from build123d import *

# Parameters (mm, degrees)
SKETCH_1_W          = 45
SKETCH_1_H          = 247
EXTRUDE_1_DEPTH     = 6
CUT_EXTRUDE_1_DEPTH = 249.095243808
M3X0_51_D           = 2.5
M3X0_51_DEPTH       = 8.5
M3X0_51_TIP         = 0.751075774
M3X0_52_D           = 2.5
M3X0_52_DEPTH       = 8.5
M3X0_52_TIP         = 0.751075774


with BuildPart() as part:
    # Эскиз1 → Бобышка-Вытянуть1 (new body)
    with BuildSketch(Plane(origin=(0, 0, 0), x_dir=(1, 0, 0), z_dir=(0, 1, 0))):
        with Locations((0, -123.5)):
            Rectangle(SKETCH_1_W, SKETCH_1_H)
    extrude(amount=EXTRUDE_1_DEPTH)

    # Эскиз2 → Вырез-Вытянуть1 (cut, through all)
    with BuildSketch(Plane(origin=(0, 6, 0), x_dir=(1, 0, 0), z_dir=(0, 1, 0))):
        with BuildLine():
            Line((-10.274368671, -73.5), (-10.274368671, -173.5))
            ThreePointArc((-10.274368671, -173.5), (-12.374368671, -175.6), (-14.474368671, -173.5))
            Line((-14.474368671, -173.5), (-14.474368671, -73.5))
            ThreePointArc((-14.474368671, -73.5), (-12.374368671, -71.4), (-10.274368671, -73.5))
        make_face()
        with BuildLine():
            Line((10.274368671, -73.5), (10.274368671, -173.5))
            ThreePointArc((10.274368671, -173.5), (12.374368671, -175.6), (14.474368671, -173.5))
            Line((14.474368671, -173.5), (14.474368671, -73.5))
            ThreePointArc((14.474368671, -73.5), (12.374368671, -71.4), (10.274368671, -73.5))
        make_face()
    extrude(amount=-CUT_EXTRUDE_1_DEPTH, mode=Mode.SUBTRACT)

    # Отверстие обработанное метчиком M3x0.51
    with Locations(Plane.XY.offset(247)):
        with Locations((-13.5, 3), (-4.5, 3), (4.5, 3), (13.5, 3)):
            Hole(M3X0_51_D / 2, depth=M3X0_51_DEPTH)
            with Locations((0, 0, -(M3X0_51_DEPTH + M3X0_51_TIP / 2))):  # 118° drill point
                Cone(0, M3X0_51_D / 2, M3X0_51_TIP, mode=Mode.SUBTRACT)

    # Отверстие обработанное метчиком M3x0.52
    with Locations(Plane(origin=(0, 0, 0), x_dir=(-1, 0, 0), z_dir=(0, 0, -1))):
        with Locations((-13.5, 3), (-4.5, 3), (4.5, 3), (13.5, 3)):
            Hole(M3X0_52_D / 2, depth=M3X0_52_DEPTH)
            with Locations((0, 0, -(M3X0_52_DEPTH + M3X0_52_TIP / 2))):  # 118° drill point
                Cone(0, M3X0_52_D / 2, M3X0_52_TIP, mode=Mode.SUBTRACT)


solid = part.part
Geometry: final body of the model. Coordinates: model frame, mm. A direction names the side the tool comes from. Round coordinates to 2 decimals unless told otherwise and drop trailing zeros. Loops run counter-clockwise (first coordinate to the right, second up) from the corner with the lowest first, then second, coordinate; pieces in that order, holes last. Notation, with made-up numbers: (89, 40.5) - (148, 40.5) arc R20 ccw to (148, 61.5) - close; hole circle Ø9 at (-5.5, -34.75). An arc over 180 degrees is marked (long way). Write each question's results on one line, items separated by ' | '. Start each with the question number.
1) Mould query, pull axis X, two halves, no side actions, for faces 1 (the face through (-14.474, 3, 124)), 2 (the face through (22.5, 3, 125)), 3 (the face through (-22.5, 3, 125)), 4 (the face through (0, 3, 0)). Classes: released by +X, released by -X, zero draft, split by the parting line, or undercut.
2) First-contact query: P1, Ø1.5, axis at x = -13.5, y = 3, coming from the -Z side; P2, Ø2, axis at x = -13.5, y = 3, coming from the -Z side; P3, Ø2, axis at x = -4.5, y = 3, coming from the +Z side. Flat tips, straight axial feed; report the tip coordinate or a pass-through.
3) Line query: probe 1 along X at (y, z) = (2.45, 144); probe 2 along X at (y, z) = (3, 6.25); probe 3 along Z at (x, y) = (-12, 4.8). Output: solid intervals per line, ascending. Write a range as [from, to].
4) Cut plane A-A on z = 149.5. Return loops of the section in (x, y), then the cut area to 3 significant figures.
5) Access query for faces 5 (the face through (14.474, 3, 124)), 6 (the face through (0, 0, 122)). Directions: +Z, -Z, +X, -X, +Y, -Y. A direction counts if a zero-diameter tool reaches every point of the face in a straight line with its end or side. Return the directions, or none.
Verdict:
1) face 1: undercut | face 2: released by +X | face 3: released by -X | face 4: zero draft
2) P1: stops at z = 8.8 | P2: stops at z = 8.65 | P3: stops at z = 238.35
3) probe 1: x = [-22.5, -14.47], [-10.27, 10.27], [14.47, 22.5] | probe 2: x = [-22.5, -14.75], [-12.25, -5.75], [-3.25, 3.25], [5.75, 12.25], [14.75, 22.5] | probe 3: z = [0, 71.43], [175.57, 247]
4) outline: (-22.5, 0) - (-14.47, 0) - (-14.47, 6) - (-22.5, 6) - close; (-10.27, 0) - (10.27, 0) - (10.27, 6) - (-10.27, 6) - close; (14.47, 0) - (22.5, 0) - (22.5, 6) - (14.47, 6) - close | area: 220 mm2
5) face 5: +Y, -Y | face 6: +Z, -Z, +X, -X, -Y
